```python
from build123d import *

# Parameters (mm, degrees)
PAD_DEPTH       = 8
SKETCH001_R     = 1.5
POCKET_DEPTH    = 14
SKETCH002_W     = 1
SKETCH002_H     = 10
POCKET001_DEPTH = 5


with BuildPart() as part:
    # Sketch → Pad (new body)
    with BuildSketch(Plane.XZ):
        Polygon((-15, -2), (10, -2), (10, 0), (2, 0), (2, 9.9), (10, 9.9), (10, 10.9), (2, 10.9), (2, 21.6), (10, 21.6), (10, 22.6), (2, 22.6), (2, 29.6), (0, 29.6), (0, 0), (-15, 0), align=None)
    extrude(amount=PAD_DEPTH)

    # Sketch001 → Pocket (cut)
    with BuildSketch(Plane(origin=(0, 0, 22.6), x_dir=(-1, 0, 0), z_dir=(0, 0, 1))):
        with Locations((-6.5, 4)):
            Circle(SKETCH001_R)
    extrude(amount=-POCKET_DEPTH, mode=Mode.SUBTRACT)

    # Sketch002 → Pocket001 (cut)
    with BuildSketch(Plane(origin=(2, 0, 0), x_dir=(0, 0, 1), z_dir=(1, 0, 0))):
        with Locations((27.1, 0.5)):
            Rectangle(SKETCH002_W, SKETCH002_H)
        with Locations((4.24, 0.5)):
            Rectangle(SKETCH002_W, SKETCH002_H)
    extrude(amount=-POCKET001_DEPTH, mode=Mode.SUBTRACT)


solid = part.part
```
Can you work these out from the model? Positions are in its coordinate system, mm. A direction names the side the tool comes from. Coordinates: 2 decimals unless noted, no trailing zeros. Loops run counter-clockwise (first coordinate to the right, second up) from the corner with the lowest first, then second, coordinate; pieces in that order, holes last.
1) Imagine slicing it at A-A on x = 3.25. List the corners of the cut face in (y, z) for me, plus the area to 3 significant figures.
2) Imagine slicing it at D-D on y = -1.25. List the corners of the cut face in (x, z) for me, plus the area to 3 significant figures.
3) Imagine slicing it at C-C on x = 6.5. List the corners of the cut face in (y, z) for me, plus the area to 3 significant figures.
4) For pin 1 (2 mm diameter, centred on y = -2, z = 16, fed in from -X); pin 2 (2.5 mm diameter, centred on x = 6.5, y = -4, fed in from +Z); pin 3 (1.5 mm diameter, centred on x = 5, y = -6.5, fed in from +Z), each with a flat end and sliding along its axis, tell me the tip position at first contact or that it passes through.
5) Which directions (+Z, -Z, +X, -X, +Y, -Y) give clear straight access to the entire face, cutting with the end or side of a thin tool? Please do faces 1 (the flat face through (5, -3, 22.6)), 2 (the cylindrical face through (8, -4.07, 10.41)), 3 (the flat face through (1, -3, 27.6)).
6) Imagine slicing it at B-B on y = -4. State how many separate pieces and enclosed holes the cut face has, plus the area to 3 significant figures.
7) I need wall thicknesses on probe 1 along Z at (x, y) = (2.25, -3.25); probe 2 along X at (y, z) = (-4, 10.7); probe 3 along Y at (x, z) = (6.5, 22.3). Which ranges of each line are inside material? Lowest first, please.
8) Thinking about a two-plate mould opening in Z: for faces 4 (the flat face through (2, -4, 5)), 5 (the flat face through (1, -4, 29.6)), 6 (the flat face through (0.2, -8, 8)), which applies, pulls with the +Z half, pulls with the -Z half, needs draft (parallel to the pull), parting line crosses it, or undercut?
Completed:
1. outline: (-8, -2) - (0, -2) - (0, 0) - (-8, 0) - close; (-8, 9.9) - (0, 9.9) - (0, 10.9) - (-8, 10.9) - close; (-8, 21.6) - (0, 21.6) - (0, 22.6) - (-8, 22.6) - close
1. area: 32.0 mm2
2. outline: (-15, -2) - (10, -2) - (10, 0) - (2, 0) - (2, 3.74) - (0, 3.74) - (0, 0) - (-15, 0) - close; (0, 4.74) - (2, 4.74) - (2, 9.9) - (10, 9.9) - (10, 10.9) - (2, 10.9) - (2, 21.6) - (10, 21.6) - (10, 22.6) - (2, 22.6) - (2, 26.6) - (0, 26.6) - close; (0, 27.6) - (2, 27.6) - (2, 29.6) - (0, 29.6) - close
2. area: 121 mm2
3. outline: (-8, -2) - (0, -2) - (0, 0) - (-8, 0) - close; (-8, 9.9) - (-5.5, 9.9) - (-5.5, 10.9) - (-8, 10.9) - close; (-8, 21.6) - (-5.5, 21.6) - (-5.5, 22.6) - (-8, 22.6) - close; (-2.5, 9.9) - (0, 9.9) - (0, 10.9) - (-2.5, 10.9) - close; (-2.5, 21.6) - (0, 21.6) - (0, 22.6) - (-2.5, 22.6) - close
3. area: 26.0 mm2
4. pin 1: stops at x = 0
4. pin 2: stops at z = 0
4. pin 3: stops at z = 22.6
5. face 1: +Z, +X, +Y, -Y
5. face 2: +Z
5. face 3: +X, -X, +Y
6. separate pieces: 5
6. enclosed holes: 0
6. area: 115 mm2
7. probe 1: z = -2 to 0, 9.9 to 10.9, 21.6 to 22.6
7. probe 2: x = 0 to 5, 8 to 10
7. probe 3: y = -8 to -5.5, -2.5 to 0
8. face 4: undercut
8. face 5: pulls with the +Z half
8. face 6: needs draft
